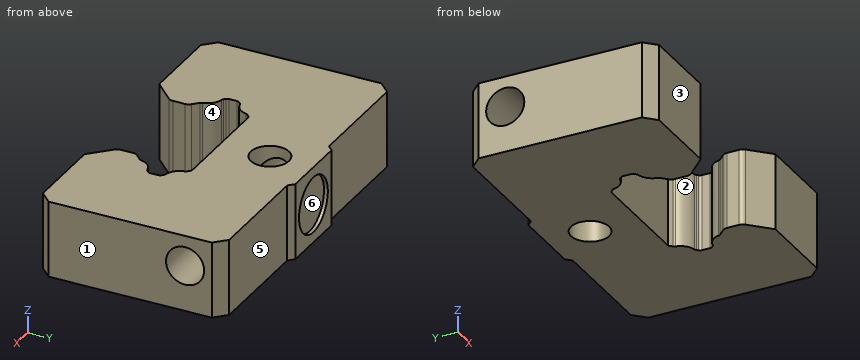
from build123d import *

# Parameters (mm, degrees)
ENDCAP_1_DEPTH                  = 10
TAP_DRILL_FOR_M6X1_0_TAP1_D     = 5
TAP_DRILL_FOR_M6X1_0_TAP1_DEPTH = 12.5
TAP_DRILL_FOR_M6X1_0_TAP1_TIP   = 1.301417626
TAP_DRILL_FOR_M6X1_0_TAP2_D     = 5
SKETCH9_R                       = 3.65
CUT_EXTRUDE1_DEPTH              = 0.5


with BuildPart() as part:
    # Sketch3 → Endcap 1 (new body)
    with BuildSketch(Plane.XY):
        with BuildLine():
            Line((-7.230720611, 12.9), (7.230720611, 12.9))
            Line((7.230720611, 12.9), (7.647672674, 12.483047938))
            ThreePointArc((7.647672674, 12.483047938), (7.736182466, 12.363118479), (7.785406885, 12.222427275))
            ThreePointArc((7.785406885, 12.222427275), (8.344607784, 11.164307384), (9.402727675, 10.605106485))
            ThreePointArc((9.402727675, 10.605106485), (9.54341888, 10.555882066), (9.663348338, 10.467372274))
            Line((9.663348338, 10.467372274), (9.853553391, 10.277167221))
            ThreePointArc((9.853553391, 10.277167221), (9.961939766, 10.114955546), (10, 9.92361383))
            Line((10, 9.92361383), (10, 8.86638617))
            ThreePointArc((10, 8.86638617), (9.961939766, 8.675044454), (9.853553391, 8.512832779))
            Line((9.853553391, 8.512832779), (9.675343394, 8.334622782))
            ThreePointArc((9.675343394, 8.334622782), (9.554347216, 8.245550888), (9.412352167, 8.19644607))
            ThreePointArc((9.412352167, 8.19644607), (8.344607784, 7.635448616), (7.783610331, 6.567704234))
            ThreePointArc((7.783610331, 6.567704234), (7.734505512, 6.425709184), (7.645433618, 6.304713007))
            Line((7.645433618, 6.304713007), (6.892893219, 5.552172608))
            ThreePointArc((6.892893219, 5.552172608), (6.676120468, 5.227749259), (6.6, 4.845065826))
            Line((6.6, 4.845065826), (6.6, 3.284934173))
            ThreePointArc((6.6, 3.284934173), (6.676120468, 2.902250741), (6.892893219, 2.577827392))
            Line((6.892893219, 2.577827392), (9.470720611, 0))
            Line((9.470720611, 0), (19.9998779, 0))
            Line((19.9998779, 0), (21.5, 1.5))
            Line((21.5, 1.5), (21.5, 22.9))
            Line((21.5, 22.9), (20.0001221, 24.4))
            Line((20.0001221, 24.4), (5.3001221, 24.4))
            Line((5.3001221, 24.4), (4.6001221, 25.1))
            Line((4.6001221, 25.1), (-4.5998779, 25.1))
            Line((-4.5998779, 25.1), (-5.2998779, 24.4))
            Line((-5.2998779, 24.4), (-19.9998779, 24.4))
            Line((-19.9998779, 24.4), (-21.5, 22.8997558))
            Line((-21.5, 22.8997558), (-21.5, 1.5))
            Line((-21.5, 1.5), (-19.9998779, 0))
            Line((-19.9998779, 0), (-9.470720611, 0))
            Line((-9.470720611, 0), (-6.892893219, 2.577827392))
            ThreePointArc((-6.892893219, 2.577827392), (-6.676120468, 2.902250741), (-6.6, 3.284934173))
            Line((-6.6, 3.284934173), (-6.6, 4.845065826))
            ThreePointArc((-6.6, 4.845065826), (-6.676120468, 5.227749259), (-6.892893219, 5.552172608))
            Line((-6.892893219, 5.552172608), (-7.645433618, 6.304713006))
            ThreePointArc((-7.645433618, 6.304713006), (-7.734505512, 6.425709184), (-7.783610331, 6.567704233))
            ThreePointArc((-7.783610331, 6.567704233), (-8.344607784, 7.635448616), (-9.412352167, 8.19644607))
            ThreePointArc((-9.412352167, 8.19644607), (-9.554347216, 8.245550888), (-9.675343394, 8.334622782))
            Line((-9.675343394, 8.334622782), (-9.853553391, 8.512832779))
            ThreePointArc((-9.853553391, 8.512832779), (-9.961939766, 8.675044454), (-10, 8.86638617))
            Line((-10, 8.86638617), (-10, 9.92361383))
            ThreePointArc((-10, 9.92361383), (-9.961939766, 10.114955546), (-9.853553391, 10.277167221))
            Line((-9.853553391, 10.277167221), (-9.663348338, 10.467372274))
            ThreePointArc((-9.663348338, 10.467372274), (-9.543418879, 10.555882066), (-9.402727675, 10.605106485))
            ThreePointArc((-9.402727675, 10.605106485), (-8.344607784, 11.164307384), (-7.785406885, 12.222427275))
            ThreePointArc((-7.785406885, 12.222427275), (-7.736182466, 12.363118479), (-7.647672674, 12.483047938))
            Line((-7.647672674, 12.483047938), (-7.230720611, 12.9))
        make_face()
    extrude(amount=ENDCAP_1_DEPTH)

    # Tap Drill for M6x1.0 Tap1
    with Locations(Plane.XY.offset(10)):
        with Locations((0, 19.4)):
            Hole(TAP_DRILL_FOR_M6X1_0_TAP1_D / 2, depth=TAP_DRILL_FOR_M6X1_0_TAP1_DEPTH)
            with Locations((0, 0, -(TAP_DRILL_FOR_M6X1_0_TAP1_DEPTH + TAP_DRILL_FOR_M6X1_0_TAP1_TIP / 2))):  # 125° drill point
                Cone(0, TAP_DRILL_FOR_M6X1_0_TAP1_D / 2, TAP_DRILL_FOR_M6X1_0_TAP1_TIP, mode=Mode.SUBTRACT)

    # Tap Drill for M6x1.0 Tap2 (through all)
    with Locations(Plane(origin=(21.5, 0, 0), x_dir=(0, 0, -1), z_dir=(1, 0, 0))):
        with Locations((-6, 19.4)):
            Hole(TAP_DRILL_FOR_M6X1_0_TAP2_D / 2)

    # Sketch9 → Cut-Extrude1 (cut)
    with BuildSketch(Plane(origin=(0, 25.1, 0), x_dir=(1, 0, 0), z_dir=(0, 1, 0))):
        with Locations(Location((0.0001221, -5, 0), (0, 0, 270))):
            Circle(SKETCH9_R)
    extrude(amount=-CUT_EXTRUDE1_DEPTH, mode=Mode.SUBTRACT)


solid = part.part
Verification items for the finished model (mm, model axes). Face numbers are marked on the shaded views. A direction names the side the tool comes from. Coordinates: 2 decimals unless noted, no trailing zeros. Order: outer loops, then holes, each group sorted by start corner. A loop starts at its lowest first (then second) coordinate and runs counter-clockwise, first axis right, second up. Notation, with made-up numbers: (7, -10) -> (30, -10) arc R28 cw to (30, 11) -> close; hole circle Ø3 at (89.5, 88.25). An arc over 180 degrees is marked (long way). Use CSV: the item, a comma, the result in double quotes. Start each with the question number.
Q1. Thickness scan on line 1 along Y through (x, z) = (0, 3.5); line 2 along X through (y, z) = (4.25, 4); line 3 along Y through (x, z) = (16, 6). Record the ranges inside material, lowest first.
Q2. Section check A-A, the plane y = 3.75. Record the cut outline in (x, z), and give its area (3 significant figures).
Q3. Draft check along Y on the marked faces 1, 2 and 3. Enter one of: +Y half, -Y half, draft (parallel to the pull), parting line (faces both ways), or undercut.
Q4. Section check C-C, the plane x = 12. Record the cut outline in (y, z).
Q5. Tool access check on the marked faces 4, 5 and 6. Record the directions out of +Z, -Z, +X, -X, +Y, -Y that give a thin tool (end or side, any length) a straight path to the whole face; none if there is none.
Q6. Section check B-B, the plane y = 19.4. Record the cut outline in (x, z).
Q7. Depth check by flat-ended pin: P1, Ø5, axis at x = 10, z = 7.5, coming from the +Y side; P2, Ø5, axis at x = 8, z = 2, coming from the -Y side. Enter the tip coordinate at first touch or a pass-through.
Q8. Section check D-D, the plane x = -2. Record the cut outline in (y, z).
Returned:
1,line 1,"y = 12.9 to 16.9, 21.9 to 24.6"
1,line 2,"x = -21.5 to -6.6, 6.6 to 21.5"
1,line 3,"y = 0 to 16.9, 21.9 to 24.4"
2,outline,"(-21.5, 0) -> (-6.6, 0) -> (-6.6, 10) -> (-21.5, 10) -> close; (6.6, 0) -> (21.5, 0) -> (21.5, 10) -> (6.6, 10) -> close"
2,area,"298 mm^2"
3,face 1,"draft"
3,face 2,"undercut"
3,face 3,"-Y half"
4,outline,"(0, 0) -> (24.4, 0) -> (24.4, 10) -> (0, 10) -> close; hole circle Ø5 at (19.4, 6)"
5,face 4,"+Z, -Z"
5,face 5,"+Z, -Z, +X, +Y"
5,face 6,"+Y"
6,outline,"(-21.5, 0) -> (-2.5, 0) -> (-2.5, 3.5) -> (-21.5, 3.5) -> close; (-21.5, 8.5) -> (-2.5, 8.5) -> (-2.5, 10) -> (-21.5, 10) -> close; (2.5, 0) -> (21.5, 0) -> (21.5, 3.5) -> (2.5, 3.5) -> close; (2.5, 8.5) -> (21.5, 8.5) -> (21.5, 10) -> (2.5, 10) -> close"
7,P1,"stops at y = 24.4"
7,P2,"stops at y = 0"
8,outline,"(12.9, 0) -> (17.9, 0) -> (17.9, 4) arc R2.5 cw to (17.9, 8) -> (17.9, 10) -> (12.9, 10) -> close; (20.9, 0) -> (25.1, 0) -> (25.1, 1.95) -> (24.6, 1.95) -> (24.6, 8.05) -> (25.1, 8.05) -> (25.1, 10) -> (20.9, 10) -> (20.9, 8) arc R2.5 cw to (20.9, 4) -> close"
